Autodesk Inventor part; units mm, degrees
ref_plane "YZ Plane" through (0, 0, 0) normal (1, 0, 0) x (0, 1, 0)
ref_plane "XZ Plane" through (0, 0, 0) normal (0, 1, 0) x (-1, 0, 0)
ref_plane "XY Plane" through (0, 0, 0) normal (0, 0, 1) x (1, 0, 0)
sketch "Boceto1" plane through (0, 0, 0) normal (0, 1, 0) x (-1, 0, 0)
  circle A0 centre (0, 0) radius 7
  dimension "d0" = 14
extrude "Extrusión1" add sketch "Boceto1" along normal blind 7.7
sketch "Boceto2" plane through (0, 7.7, 0) normal (0, 1, 0) x (1, 0, 0)
  circle A0 centre (0, 0) radius 6.85
  dimension "d3" = 13.7
extrude "Extrusión2" cut sketch "Boceto2" against normal blind 7.6
sketch "Boceto3" plane through (0, 0, 0) normal (0, -1, 0) x (1, 0, 0)
  circle A0 centre (0, 0) radius 2.5
  dimension "d6" = 5
extrude "Extrusión3" add sketch "Boceto3" along normal blind 10
sketch "Boceto4" plane through (0, -10, 0) normal (0, -1, 0) x (1, 0, 0)
  arc A0 (-1.9, 1.6248) -> (-1.9, -1.6248) centre (0, 0) ccw
  arc A1 (1.9, -1.6248) -> (1.9, 1.6248) centre (0, 0) ccw
  circle A2 centre (0, 0) radius 2.5
  line L0 (0, 0) -> (1.9, 0)
  line L1 (-1.9, 0) -> (-1.9, 1.6248)
  line L2 (-1.9, 0) -> (-1.9, -1.6248)
  line L3 (1.9, 0) -> (1.9, 1.6248)
  line L4 (1.9, 0) -> (1.9, -1.6248)
  point P0 (-1.6248, 1.9)
  point P1 (-1.6248, -1.9)
  point P2 (1.6248, -1.9)
  point P3 (1.6248, 1.9)
extrude "Extrusión4" cut sketch "Boceto4" against normal blind 10 contours L1 L2 A0 | A1 L4 L3
sketch "Boceto6" plane through (1.9, -10, 1.6248) normal (1, 0, 0) x (0, 0, -1)
  line L0 (1.6248, 10) -> (1.6248, 8.6)
  circle A0 centre (1.6248, 4.3) radius 4.3
  dimension "d18" = 1.4
  dimension "d20" = 8.6
extrude "Extrusión5" add sketch "Boceto6" against normal blind 3.8
sketch "Boceto7" plane through (1.9, -10, 1.6248) normal (1, 0, 0) x (0, 0, -1)
  arc A0 (-0.8752, 0.8014) -> (4.1248, 0.8014) centre (1.6248, 4.3) ccw
  line L0 (3.2496, 0) -> (4.1248, 0)
  line L1 (-0.8752, 0) -> (0, 0)
  line L2 (4.1248, 0.8014) -> (4.1248, 0)
  line L3 (4.1248, 0.8014) -> (4.1248, 0)
  line L4 (-0.8752, 0.8014) -> (-0.8752, 0)
  line L5 (-0.8752, 0.8014) -> (-0.8752, 0)
  arc A1 (-0.8752, 0.8014) -> (4.1248, 0.8014) centre (1.6248, 4.3) ccw
  line L6 (-0.8752, 0) -> (1.6248, 0)
  line L7 (3.2496, 0) -> (0, 0)
  line L8 (1.6248, 0) -> (4.1248, 0)
  point P0 (1.6248, 10)
extrude "Extrusión6" cut sketch "Boceto7" against normal blind 3.8
sketch "Boceto8" plane through (-1.9, 0, -1.6248) normal (-1, 0, 0) x (0, 0, 1)
  circle A0 centre (1.6248, -5.7) radius 2.55
  point P0 (1.6248, 0)
  dimension "d28" = 5.1
extrude "Extrusión7" cut sketch "Boceto8" against normal blind 3.8
fillet "Empalme1" radius 0.02 2 edges at (1.9, -5.7, -2.55) (-1.9, -5.7, -2.55)
properties part number "Conexion_inferior"
The model under review builds one solid part; all positions refer to its coordinate system, in mm. A direction names the side the tool comes from. Round coordinates to 2 decimals unless told otherwise and drop trailing zeros. Order: outer loops, then holes, each group sorted by start corner. A loop starts at its lowest first (then second) coordinate and runs counter-clockwise, first axis right, second up. Notation, with made-up numbers: (5, 50.25) -> (13, 50.25) arc R15 cw to (13, 79.25) -> close; hole circle Ø3 at (88, -40). An arc over 180 degrees is marked (long way). Write item = value, one per line. Start each with the question number.
Item 1: Consider section D-D on x = -4. Write out the cut boundary in (y, z), plus the area to 3 significant figures.
Item 2: Clearance check with flat-ended pins moving along their axes: pin 1 Ø4 at (y, z) = (-5.7, 0) entering from +X; pin 2 Ø4 at (x, y) = (0.5, -7.5) entering from +Z; pin 3 Ø4 at (x, z) = (1, -2.5) entering from +Y; pin 4 Ø4.5 at (y, z) = (-5.5, -2) entering from -X. State where each tip first meets the part, or that it passes through.
Item 3: Mouldability with a two-part tool opening along X and no side actions: class faces 6 (the face through (-0.03, -7.96, 1.18)), 7 (the face through (-0.89, 3.95, -6.79)), 8 (the face through (1.9, -3.8, 2)) as released by +X, released by -X, zero draft, split by the parting line, or undercut.
Item 4: For faces 1 (the face through (-1.9, -2.8, -0.1)), 2 (the face through (0, 0.1, 0)), 3 (the face through (-6.677, 3.796, -2.103)), 4 (the face through (0, -1.1, -2.5)), 5 (the face through (0, -1.1, 2.5)), list the 3-axis set-ups (+Z, -Z, +X, -X, +Y, -Y) from which the entire face can be reached by the end or side of a thin tool; tool diameter is ignored.
Item 5: For line 1 along Z through (x, y) = (-1.75, 5); line 2 along X through (y, z) = (-2, -1.75); line 3 along X through (y, z) = (3, -1), list the stretches that pass through material, from the lowest coordinate up.
Item 6: Consider section C-C on z = 4. Write out the cut boundary in (x, y), plus the area to 3 significant figures.
Conclusion:
q1.outline = (0, -5.74) -> (7.7, -5.74) -> (7.7, -5.56) -> (0.1, -5.56) -> (0.1, 5.56) -> (7.7, 5.56) -> (7.7, 5.74) -> (0, 5.74) -> close
q1.area = 3.94 mm2
q2.pin_1 = through
q2.pin_2 = 4.3
q2.pin_3 = 0.1
q2.pin_4 = -1.9
q3.face_6 = zero draft
q3.face_7 = undercut
q3.face_8 = released by +X
q4.face_1 = +Z, -Z, -X, -Y
q4.face_2 = +Y
q4.face_3 = +Y, -Y
q4.face_4 = -Z
q4.face_5 = +Z
q5.line_1 = -6.78 to -6.62, 6.62 to 6.78
q5.line_2 = -1.9 to 1.9
q5.line_3 = -6.93 to -6.78, 6.78 to 6.93
q6.outline = (-5.74, 0) -> (5.74, 0) -> (5.74, 7.7) -> (5.56, 7.7) -> (5.56, 0.1) -> (-5.56, 0.1) -> (-5.56, 7.7) -> (-5.74, 7.7) -> close; (-1.9, -7.28) -> (1.9, -7.28) -> (1.9, -4.12) -> (-1.9, -4.12) -> close
q6.area = 15.9 mm2
